CAD build for the part. Positions are in the model's coordinates, mm. A direction names the side the tool comes from. Give positions to 0.01 mm unless a question says otherwise; leave off trailing zeros. Order: outer loops, then holes, each group sorted by start corner. A loop starts at its lowest first (then second) coordinate and runs counter-clockwise, first axis right, second up.
Item 1: Wall check: L1, parallel to Z at x = 16, y = -3.25; L2, parallel to Y at x = -76.5, z = 48.5; L3, parallel to X at y = -3, z = 5. Give the ranges that are in metal, low to high.
Item 2: Band-saw the part on A-A on y = -1.75. Give the cut face in (x, z).
Item 3: Flat gauge pins, fed straight in: P1, Ø4.5, axis at x = 17.5, y = -2.5, coming from the +Z side; P2, Ø3, axis at x = -2.5, y = -3, coming from the -Z side; P3, Ø2, axis at y = -2.5, z = 3.5, coming from the -X side. Where does each tip first touch, or does it go through?
Item 4: Which spindle directions (+Z, -Z, +X, -X, +Y, -Y) get a long thin tool onto all of the face, cutting with end or side? Do faces 1 (the cylindrical face through (-81.972, -2.028, 41.094)), 2 (the flat face through (-94, -2, 0)), 3 (the flat face through (1, -2, -52.5)). Say none if no direction does.
Item 5: Band-saw the part on B-B on z = 3. Give the cut face in (x, y), plus the area to 3 significant figures.
Autodesk Inventor part; units mm, degrees
ref_plane "YZ Plane" through (0, 0, 0) normal (1, 0, 0) x (0, 1, 0)
ref_plane "XZ Plane" through (0, 0, 0) normal (0, 1, 0) x (-1, 0, 0)
ref_plane "XY Plane" through (0, 0, 0) normal (0, 0, 1) x (1, 0, 0)
sketch "Sketch2" plane through (0, 0, 0) normal (0, 1, 0) x (-1, 0, 0)
  line L0 (-100, 58.5) -> (-100, -58.5)
  line L1 (-100, -58.5) -> (100, -58.5)
  line L2 (100, -58.5) -> (100, 58.5)
  line L3 (100, 58.5) -> (-100, 58.5)
  point P0 (0, 0)
  point P1 (100, 0)
  dimension "d0" = 117
  dimension "d1" = 200
  dimension "d2" = 58.5
  dimension "d3" = 100
extrude "Extrusion1" add sketch "Sketch2" along normal blind 5
sketch "Sketch3" plane through (0, 0, 0) normal (0, -1, 0) x (1, 0, 0)
  line L0 (94, -52.5) -> (-94, -52.5)
  line L1 (-94, -52.5) -> (-94, 52.5)
  line L2 (-94, 52.5) -> (94, 52.5)
  line L3 (94, 52.5) -> (94, -52.5)
  line L4 (100, -58.5) -> (-100, -58.5)
  line L5 (-100, 58.5) -> (100, 58.5)
  line L6 (-100, -58.5) -> (-100, 58.5)
  line L7 (100, 58.5) -> (100, -58.5)
  point P0 (0, 0)
  dimension "d6" = 6
  dimension "d7" = 6
  dimension "d8" = 6
  dimension "d9" = 6
extrude "Extrusion2" add sketch "Sketch3" along normal blind 4 contours L0 L1 L2 L3
fillet "Fillet1" radius 40 4 edges at (94, -2, 52.5) (-94, -2, 52.5) (-94, -2, -52.5) (94, -2, -52.5)
properties part number "clip-cover"
The answers:
1. L1: z = -52.5 to 52.5
1. L2: y = 0 to 5
1. L3: x = -94 to 94
2. outline: (-94, -12.5) arc R40 ccw to (-54, -52.5) - (54, -52.5) arc R40 ccw to (94, -12.5) - (94, 12.5) arc R40 ccw to (54, 52.5) - (-54, 52.5) arc R40 ccw to (-94, 12.5) - close
3. P1: stops at z = 52.5
3. P2: stops at z = -52.5
3. P3: stops at x = -94
4. face 1: +Z, -X, -Y
4. face 2: +Z, -Z, -X, -Y
4. face 3: -Z, +X, -X, -Y
5. outline: (-100, 0) - (-94, 0) - (-94, -4) - (94, -4) - (94, 0) - (100, 0) - (100, 5) - (-100, 5) - close
5. area: 1,750 mm2
